Answer from the drawing. Dimensions are ordinates in mm from the lowest x, y and z of the part. Give positions to 0.01 mm unless a question says otherwise; leave off trailing zeros. Loops run counter-clockwise (first coordinate to the right, second up) from the corner with the lowest first, then second, coordinate; pieces in that order, holes last.
Item 1: Section D-D, the plane y = 2.25 is taken. Give the vertices of the cut face in (x, z), and give its area (3 significant figures).
Item 2: Section A-A, the plane x = 4.5 is taken. Give the vertices of the cut face in (y, z), and give its area (3 significant figures).
Item 3: The mould has two halves that part along Y. Classify the marked faces 1, 2 and 3: pulls with the +Y half, pulls with the -Y half, needs draft (parallel to the pull), parting line crosses it, or undercut.
Item 4: Consider line 1 along Y through (x, z) = (4.5, 10.75); line 2 along Y through (x, z) = (4.5, 30.65); line 3 along Z through (x, y) = (7.75, 4.5). Determine where each line is inside the solid, lowest interval first.
Item 5: Each of these flat-tipped pins is pushed along its axis until it touches: pin 1 Ø1 at (x, y) = (3.5, 4) entering from -Z; pin 2 Ø5 at (x, z) = (1.5, 20.5) entering from -Y; pin 3 Ø2 at (y, z) = (2, 20) entering from -X; pin 4 Ø1 at (x, z) = (8, 7) entering from -Y. Where does it stop, or does it pass through?
Item 6: Section C-C, the plane z = 17.5 is taken. Give the vertices of the cut face in (x, y), and give its area (3 significant figures).
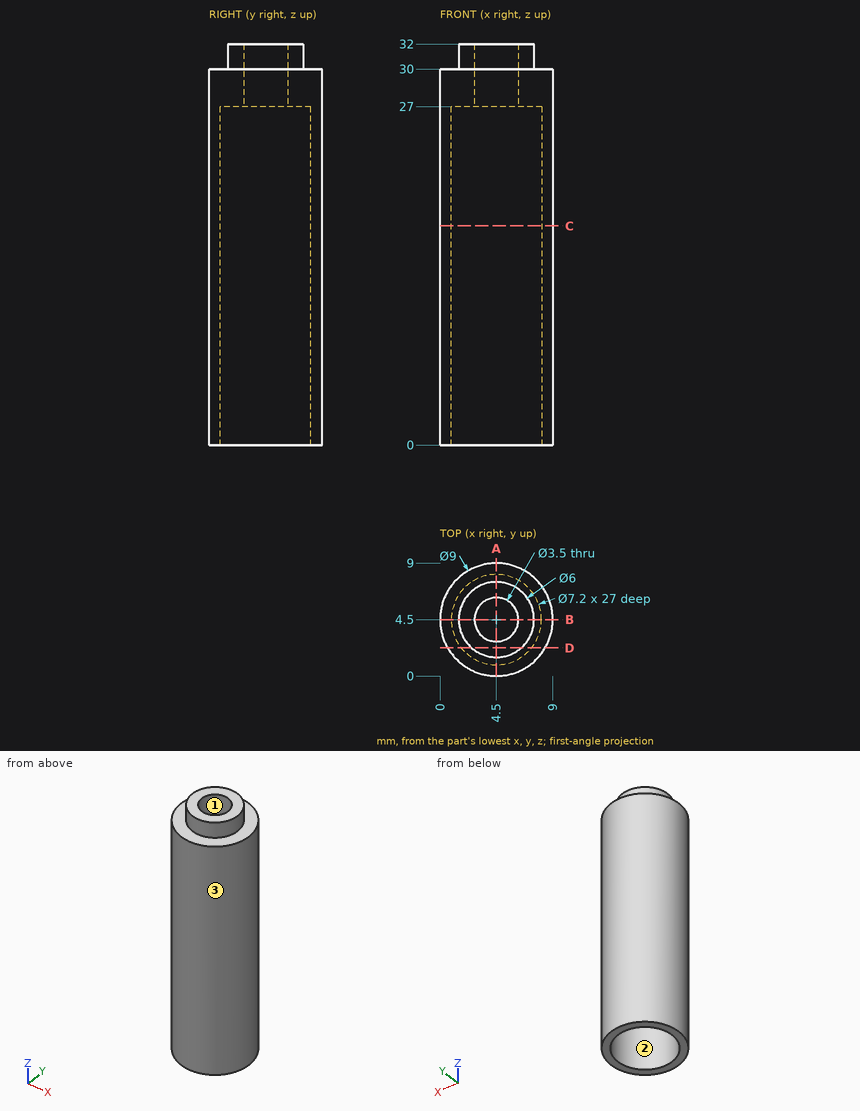
Worked answers:
1. outline: (0.6, 0) - (1.69, 0) - (1.69, 27) - (7.31, 27) - (7.31, 0) - (8.4, 0) - (8.4, 30) - (6.48, 30) - (6.48, 32) - (2.52, 32) - (2.52, 30) - (0.6, 30) - close
1. area: 90.0 mm2
2. outline: (0, 0) - (0.9, 0) - (0.9, 27) - (2.75, 27) - (2.75, 32) - (1.5, 32) - (1.5, 30) - (0, 30) - close; (6.25, 27) - (8.1, 27) - (8.1, 0) - (9, 0) - (9, 30) - (7.5, 30) - (7.5, 32) - (6.25, 32) - close
2. area: 70.1 mm2
3. face 1: undercut
3. face 2: undercut
3. face 3: parting line crosses it
4. line 1: y = 0 to 0.9, 8.1 to 9
4. line 2: y = 1.5 to 2.75, 6.25 to 7.5
4. line 3: z = 27 to 30
5. pin 1: passes through
5. pin 2: stops at y = 0.03
5. pin 3: stops at x = 0.26
5. pin 4: stops at y = 1.15
6. outline: circle Ø9 at (4.5, 4.5); hole circle Ø7.2 at (4.5, 4.5)
6. area: 22.9 mm2
